Source: three-view drawing plus pictorial views. Frame: mm from the lowest corner of the part. Give positions to 0.01 mm unless a question says otherwise; leave off trailing zeros. Loops run counter-clockwise (first coordinate to the right, second up) from the corner with the lowest first, then second, coordinate; pieces in that order, holes last. Notation, with made-up numbers: (56, -17) -> (71, -17) arc R12 cw to (71, -8) -> close; hole circle Ø8 at (42.25, -34). An arc over 180 degrees is marked (long way). Answer as a JSON object with one key per item and string values. Group by question number.
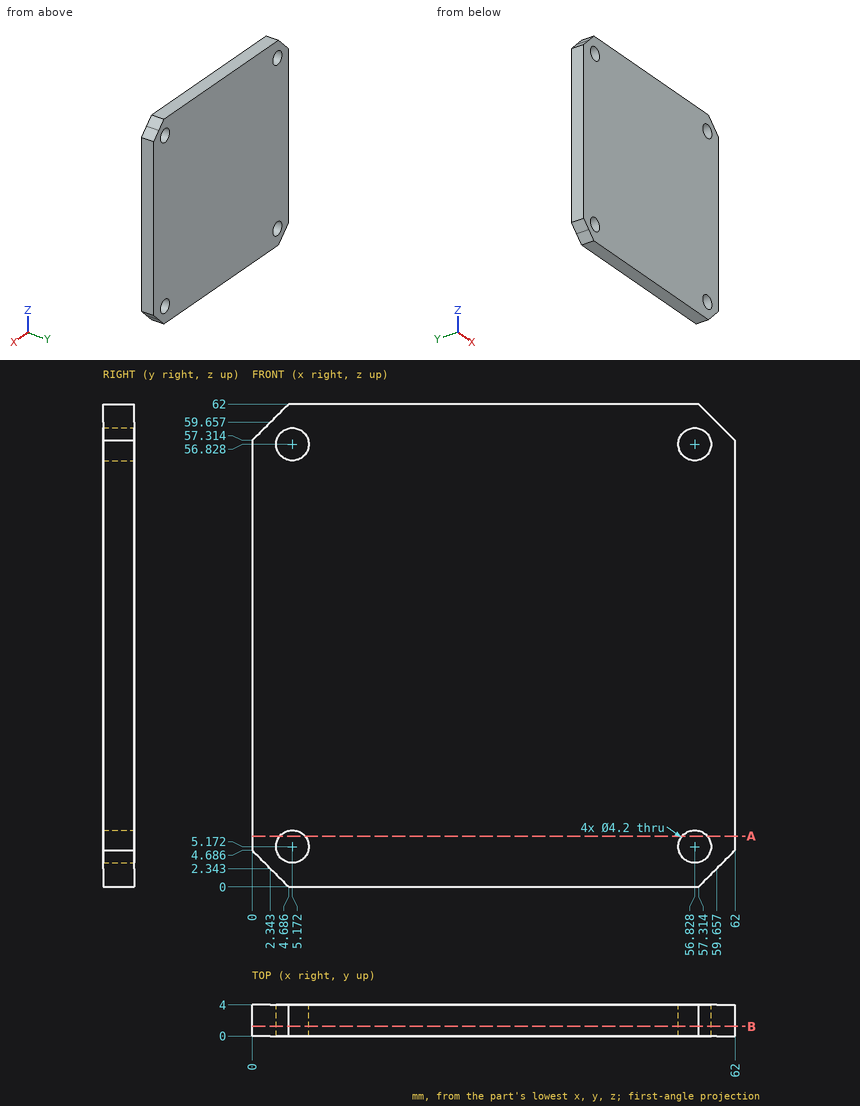
(1) Section query A-A on z = 6.5. Return the cut outline in (x, y) (1 decimal), plus the area to 3 significant figures.
(2) First-contact query: pin 1 (5.5 mm diameter, centred on x = 5.17, z = 5.17, fed in from -Y). Flat tip, straight axial feed; report the tip coordinate or a pass-through.
(3) Section query B-B on y = 1.25. Return the cut outline in (x, z), plus the area to 3 significant figures.
(4) Material intervals for line 1 (X direction, y = 2.1, z = 5) (1 decimal); line 2 (Z direction, x = 56, y = 2.5); line 3 (Z direction, x = 55.5, y = 3.25) (1 decimal), sorted ascending. Write a range as from..to.
Result:
{
 "1": {"outline": "(0, 0) -> (3.5, 0) -> (3.5, 4) -> (0, 4) -> close; (6.8, 0) -> (55.2, 0) -> (55.2, 4) -> (6.8, 4) -> close; (58.5, 0) -> (62, 0) -> (62, 4) -> (58.5, 4) -> close", "area": "222 mm²"},
 "2": {"pin 1": "y = 0"},
 "3": {"outline": "(0, 4.69) -> (2.34, 2.34) -> (4.69, 0) -> (57.31, 0) -> (59.66, 2.34) -> (62, 4.69) -> (62, 57.31) -> (59.66, 59.66) -> (57.31, 62) -> (4.69, 62) -> (2.34, 59.66) -> (0, 57.31) -> close; hole circle Ø4.2 at (5.17, 5.17); hole circle Ø4.2 at (5.17, 56.83); hole circle Ø4.2 at (56.83, 5.17); hole circle Ø4.2 at (56.83, 56.83)", "area": "3,740 mm²"},
 "4": {"line 1": "0..3.1, 7.3..54.7, 58.9..62", "line 2": "0..3.24, 7.1..54.9, 58.76..62", "line 3": "0..3.5, 6.8..55.2, 58.5..62"}
}
